from build123d import *

# Parameters (mm, degrees)
SKETCH_1_R          = 1.5
EXTRUDE_1_DEPTH     = 4
EXTRUDE_START       = -4
SKETCH_2_R          = 1.5
EXTRUDE_2_DEPTH     = 4
SKETCH_3_R          = 1.5
CUT_EXTRUDE_1_DEPTH = 10


with BuildPart() as part:
    # Эскиз1 → Бобышка-Вытянуть1 (new body)
    with BuildSketch(Plane.XY):
        with BuildLine():
            ThreePointArc((14.071260881, -6.013492872), (12.319653053, -3.733490841), (9.621977893, -2.738961818))
            ThreePointArc((9.621977893, -2.738961818), (9.902389121, -1.423748614), (10.003874897, -0.082809815))
            ThreePointArc((10.003874897, -0.082809815), (12.872466462, 0.111410875), (15.195472667, 1.805571852))
            ThreePointArc((15.195472667, 1.805571852), (15.146612375, 2.177754087), (15.088637629, 2.548625862))
            ThreePointArc((15.088637629, 2.548625862), (12.382429194, 3.519694937), (9.575317452, 2.897872688))
            ThreePointArc((9.575317452, 2.897872688), (9.100156446, 4.155902197), (8.460565465, 5.338839053))
            ThreePointArc((8.460565465, 5.338839053), (10.768774621, 7.053105583), (11.807079223, 9.734236463))
            ThreePointArc((11.807079223, 9.734236463), (11.564758421, 10.020920215), (11.315478542, 10.301573893))
            ThreePointArc((11.315478542, 10.301573893), (8.513871556, 9.655402442), (6.488561375, 7.614653091))
            ThreePointArc((6.488561375, 7.614653091), (5.408688398, 8.416083426), (4.231086277, 9.065444244))
            ThreePointArc((4.231086277, 9.065444244), (5.246072926, 11.755489103), (4.67002155, 14.572349777))
            ThreePointArc((4.67002155, 14.572349777), (4.311175381, 14.68251498), (3.949734969, 14.783845))
            ThreePointArc((3.949734969, 14.783845), (1.942219856, 12.725587893), (1.341732908, 9.91383494))
            ThreePointArc((1.341732908, 9.91383494), (0, 10.004217632), (-1.341732908, 9.91383494))
            ThreePointArc((-1.341732908, 9.91383494), (-1.942219856, 12.725587893), (-3.949734969, 14.783845))
            ThreePointArc((-3.949734969, 14.783845), (-4.311175381, 14.68251498), (-4.67002155, 14.572349777))
            ThreePointArc((-4.67002155, 14.572349777), (-5.246072926, 11.755489103), (-4.231086277, 9.065444244))
            ThreePointArc((-4.231086277, 9.065444244), (-5.408688398, 8.416083426), (-6.488561375, 7.614653091))
            ThreePointArc((-6.488561375, 7.614653091), (-8.513871556, 9.655402442), (-11.315478542, 10.301573893))
            ThreePointArc((-11.315478542, 10.301573893), (-11.564758421, 10.020920215), (-11.807079223, 9.734236463))
            ThreePointArc((-11.807079223, 9.734236463), (-10.768774621, 7.053105583), (-8.460565465, 5.338839053))
            ThreePointArc((-8.460565465, 5.338839053), (-9.100156446, 4.155902197), (-9.575317452, 2.897872688))
            ThreePointArc((-9.575317452, 2.897872688), (-12.382429194, 3.519694937), (-15.088637629, 2.548625862))
            ThreePointArc((-15.088637629, 2.548625862), (-15.146612375, 2.177754087), (-15.195472667, 1.805571852))
            ThreePointArc((-15.195472667, 1.805571852), (-12.872466462, 0.111410875), (-10.003874897, -0.082809815))
            ThreePointArc((-10.003874897, -0.082809815), (-9.902389121, -1.423748614), (-9.621977893, -2.738961818))
            ThreePointArc((-9.621977893, -2.738961818), (-12.319653053, -3.733490841), (-14.071260881, -6.013492872))
            ThreePointArc((-14.071260881, -6.013492872), (-13.91952392, -6.356833577), (-13.759410906, -6.696349066))
            ThreePointArc((-13.759410906, -6.696349066), (-10.889241154, -6.865655999), (-8.371024733, -5.478167151))
            ThreePointArc((-8.371024733, -5.478167151), (-7.560683217, -6.551369301), (-6.613728339, -7.506195299))
            ThreePointArc((-6.613728339, -7.506195299), (-8.345474114, -9.801319657), (-8.586358225, -12.666370108))
            ThreePointArc((-8.586358225, -12.666370108), (-8.273084972, -12.873171495), (-7.954833402, -13.072226469))
            ThreePointArc((-7.954833402, -13.072226469), (-5.448758719, -11.662925603), (-4.080433364, -9.134245124))
            ThreePointArc((-4.080433364, -9.134245124), (-2.818513813, -9.598976524), (-1.505666768, -9.89026481))
            ThreePointArc((-1.505666768, -9.89026481), (-1.72166611, -12.757298735), (-0.375347502, -15.297764332))
            ThreePointArc((-0.375347502, -15.297764332), (0, -15.302368421), (0.375347502, -15.297764332))
            ThreePointArc((0.375347502, -15.297764332), (1.72166611, -12.757298735), (1.505666768, -9.89026481))
            ThreePointArc((1.505666768, -9.89026481), (2.818513813, -9.598976524), (4.080433364, -9.134245124))
            ThreePointArc((4.080433364, -9.134245124), (5.448758719, -11.662925603), (7.954833402, -13.072226469))
            ThreePointArc((7.954833402, -13.072226469), (8.273084972, -12.873171495), (8.586358225, -12.666370108))
            ThreePointArc((8.586358225, -12.666370108), (8.345474114, -9.801319657), (6.613728339, -7.506195299))
            ThreePointArc((6.613728339, -7.506195299), (7.560683217, -6.551369301), (8.371024733, -5.478167151))
            ThreePointArc((8.371024733, -5.478167151), (10.889241154, -6.865655999), (13.759410906, -6.696349066))
            ThreePointArc((13.759410906, -6.696349066), (13.91952392, -6.356833577), (14.071260881, -6.013492872))
        make_face()
        Circle(SKETCH_1_R, mode=Mode.SUBTRACT)
    extrude(amount=EXTRUDE_1_DEPTH)

    # Эскиз2 → Бобышка-Вытянуть2 (add)
    with BuildSketch(Plane.XY.offset(4).offset(EXTRUDE_START)):
        with BuildLine():
            Line((-13.27175932, 43.680693777), (-14.149597226, 43.649446698))
            ThreePointArc((-14.149597226, 43.649446698), (-15.542077543, 43.013723237), (-16.077185448, 41.579566593))
            Line((-16.077185448, 41.579566593), (-15.198219126, 16.886379902))
            ThreePointArc((-15.198219126, 16.886379902), (-14.029929813, 13.848310241), (-11.239138319, 12.173123678))
            Line((-11.239138319, 12.173123678), (-7.216634951, -2.042101853))
            ThreePointArc((-7.216634951, -2.042101853), (2.042101853, -7.216634951), (7.216634951, 2.042101853))
            Line((7.216634951, 2.042101853), (4.487820228, 11.685528641))
            ThreePointArc((4.487820228, 11.685528641), (2.878536468, 14.16449679), (0.150531719, 15.301628001))
            Line((0.150531719, 15.301628001), (-2.91779922, 15.593698218))
            ThreePointArc((-2.91779922, 15.593698218), (-4.851213091, 16.18881198), (-6.390589925, 17.501278571))
            ThreePointArc((-6.390589925, 17.501278571), (-11.35627908, 28.85521173), (-11.248467313, 41.247073721))
            ThreePointArc((-11.248467313, 41.247073721), (-11.662703429, 42.960565491), (-13.27175932, 43.680693777))
        make_face()
        Circle(SKETCH_2_R, mode=Mode.SUBTRACT)
    extrude(amount=EXTRUDE_2_DEPTH)

    # Эскиз3 → Вырез-Вытянуть1 (cut)
    with BuildSketch(Plane.XY.offset(4)):
        with Locations((0, 7)):
            Circle(SKETCH_3_R)
        with Locations((7, 0)):
            Circle(SKETCH_3_R)
        with Locations((0, -7)):
            Circle(SKETCH_3_R)
        with Locations((-7, 0)):
            Circle(SKETCH_3_R)
    extrude(amount=-CUT_EXTRUDE_1_DEPTH, mode=Mode.SUBTRACT)


solid = part.part
Work out the finished part from the listing and answer in its coordinate system (mm). A direction names the side the tool comes from. Coordinates: 2 decimals unless noted, no trailing zeros. Order: outer loops, then holes, each group sorted by start corner. A loop starts at its lowest first (then second) coordinate and runs counter-clockwise, first axis right, second up. Notation, with made-up numbers: (35.25, -37.75) - (39.25, -37.75) arc R26 ccw to (39.25, -15.75) - close; hole circle Ø4 at (-17, 67.5). An arc over 180 degrees is marked (long way). Put each result on its own line as item: value. Start each with the question number.
1) Find section B-B (z = 1). State how many separate pieces and enclosed holes the cut face has, plus the area to 3 significant figures.
2) For faces 4 (the cylindrical face through (1.713, -12.797, 1.972)), 5 (the cylindrical face through (1.684, 14.904, 1.972)), determine the directions among +Z, -Z, +X, -X, +Y, -Y from which every point of the face is accessible in a straight line to the end or side of a thin tool.
3) Find section C-C (y = 21). Give the vertices of the cut face in (x, z).
4) For a pull along X with two mould halves and no side action, classify faces 1 (the flat face through (-4, 8, 4)), 2 (the cylindrical face through (-15.527, 43.03, 1.972)), 3 (the flat face through (5.158, 9.318, 1.972)) as released by +X, released by -X, zero draft, split by the parting line, or undercut.
5) A flat-ended cylindrical pin translates along its axis: pin 1 (1.5 mm diameter, centred on x = -7, z = 3, fed in from +Y). Find the tip coordinate at first contact, or state that the pin passes through.
6) Find section A-A (y = 7). Give the vertices of the cut face in (x, z), plus the area to 3 significant figures.
7) Find the intervals of material crossed by line 1 (Y direction, x = 0, z = 1.35); line 2 (Y direction, x = -13, z = 2.55); line 3 (X direction, y = 8, z = 1.65), in increasing order. Write a range as from..to.
Results list:
1. separate pieces: 1
1. enclosed holes: 5
1. area: 676 mm^2
2. face 4: +Z, -Z
2. face 5: +Z, -Z, +Y
3. outline: (-15.34, 0) - (-8.55, 0) - (-8.55, 4) - (-15.34, 4) - close
4. face 1: zero draft
4. face 2: released by -X
4. face 3: undercut
5. pin 1: stops at y = 19.57
6. outline: (-10.73, 0) - (-1.5, 0) - (-1.5, 4) - (-10.73, 4) - close; (1.5, 0) - (10.73, 0) - (10.73, 4) - (1.5, 4) - close
6. area: 73.8 mm^2
7. line 1: y = -15.3..-8.5, -5.5..-1.5, 1.5..5.5, 8.5..15.32
7. line 2: y = -6.9..-4.33, 0.16..3.44, 12.92..43.67
7. line 3: x = -11.34..-1.12, 1.12..6.01, 6.72..11.34
